Study the drawing (mm; zero at the part's minimum x, y, z) and answer. A direction names the side the tool comes from. Round coordinates to 2 decimals unless told otherwise and drop trailing zeros. Loops run counter-clockwise (first coordinate to the right, second up) from the corner with the lowest first, then second, coordinate; pieces in that order, holes last. Notation, with made-up numbers: (8.25, 68) - (55.25, 68) arc R20 ccw to (55.25, 81) - close; hole circle Ø10 at (-13, 26). An arc over 180 degrees is marked (long way). Use CSV: the item, a comma, the result in double quotes. Start each with the question number.
1. Determine the mould class of the marked faces 1, 2 and 3 for opening direction X: +X half, -X half, draft (parallel to the pull), parting line (faces both ways), or undercut.
2. Given pin 1 Ø1.9 at (x, z) = (11.5, 3.5) entering from -Y; pin 2 Ø2 at (x, y) = (14.5, 32) entering from +Z; pin 3 Ø1 at (x, y) = (31.5, 9.5) entering from -Z, each flat-ended and moving along its own axis, determine where each tip first touches the part or whether it passes through.
3. A tool of negligible diameter and unlimited length cuts with its end or side. For the marked faces 4 and 5, from which of +Z, -Z, +X, -X, +Y, -Y can it reach the whole face along a straight path? Write none if from no direction.
4. Consider line 1 along X through (y, z) = (0.7, 3.5); line 2 along X through (y, z) = (5, 6.25); line 3 along X through (y, z) = (32, 9.5). Determine where each line is inside the solid, lowest interval first.
5. Find section C-C (x = 30.5). Give the vertices of the cut face in (y, z), and give its area (3 significant figures).
6. Find section A-A (x = 11.5). Give the vertices of the cut face in (y, z).
7. Find section B-B (z = 3.5). Give the vertices of the cut face in (x, y).
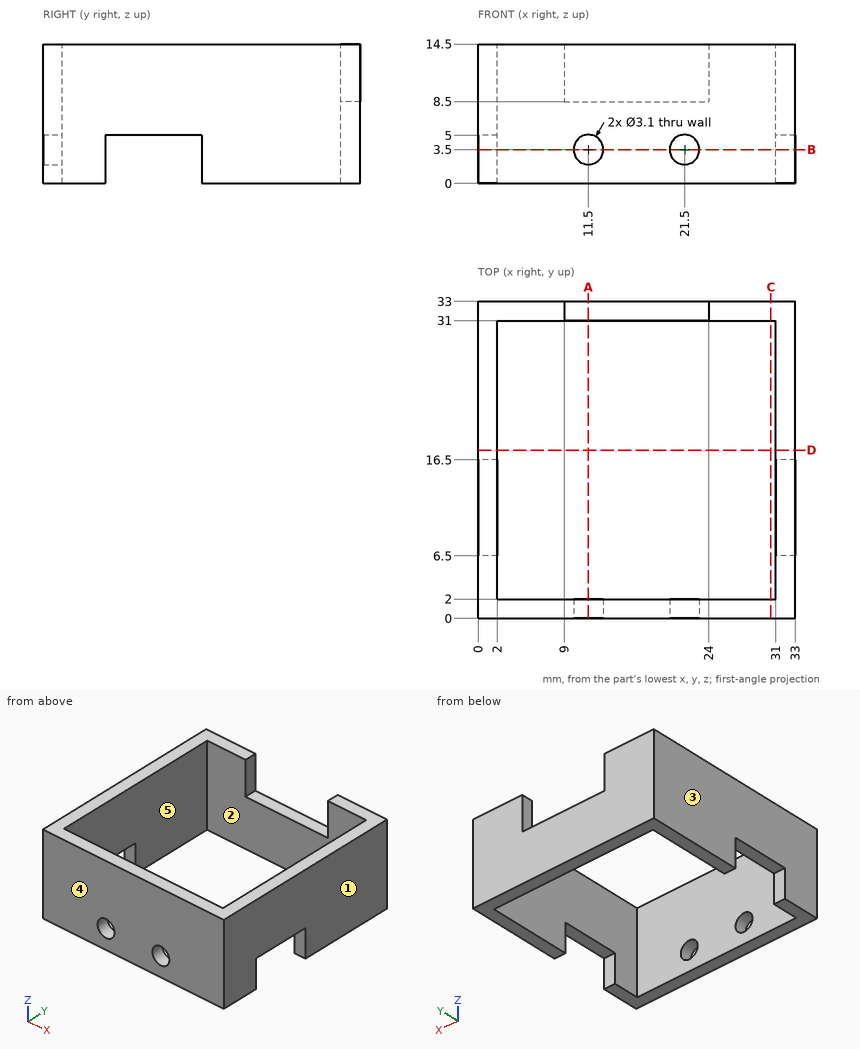
Filled sheet:
1,face 1,"+X half"
1,face 2,"undercut"
1,face 3,"-X half"
2,pin 1,"stops at y = 31"
2,pin 2,"stops at z = 8.5"
2,pin 3,"stops at z = 5"
3,face 4,"+Z, -Z, +X, -X, -Y"
3,face 5,"+Z, -Z"
4,line 1,"x = 0 to 9.95, 13.05 to 19.95, 23.05 to 33"
4,line 2,"x = 0 to 2, 31 to 33"
4,line 3,"x = 0 to 9, 24 to 33"
5,outline,"(0, 0) - (2, 0) - (2, 14.5) - (0, 14.5) - close; (31, 0) - (33, 0) - (33, 14.5) - (31, 14.5) - close"
5,area,"58.0 mm²"
6,outline,"(0, 0) - (2, 0) - (2, 1.95) - (0, 1.95) - close; (0, 5.05) - (2, 5.05) - (2, 14.5) - (0, 14.5) - close; (31, 0) - (33, 0) - (33, 8.5) - (31, 8.5) - close"
7,outline,"(0, 0) - (9.95, 0) - (9.95, 2) - (2, 2) - (2, 6.5) - (0, 6.5) - close; (0, 16.5) - (2, 16.5) - (2, 31) - (31, 31) - (31, 16.5) - (33, 16.5) - (33, 33) - (0, 33) - close; (13.05, 0) - (19.95, 0) - (19.95, 2) - (13.05, 2) - close; (23.05, 0) - (33, 0) - (33, 6.5) - (31, 6.5) - (31, 2) - (23.05, 2) - close"
